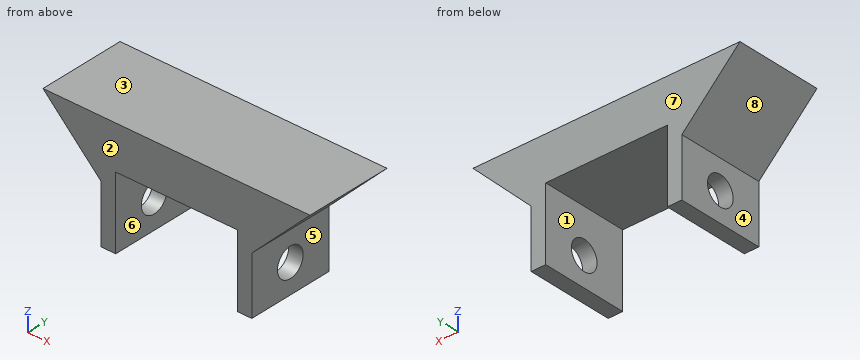
from build123d import *

# Parameters (mm, degrees)
F0_W        = 283.9974
F0_H        = 76.2
F1_DEPTH    = 50.8
F2_T1_DEPTH = 468.124487366
F3_DEPTH    = 50.8
F4_W        = 106.1974
F4_H        = 76.2
F5_DEPTH    = 63.5
F6_R        = 12.7
F7_DEPTH    = 182.3984


# Not quite as in the source:
# - a fillet or chamfer that OpenCascade refuses, or shapes differently, is made with other operations: its cross-section is extruded or revolved along the edge and cut away or added


with BuildPart() as f1:
    # F0 (on Top) → F1 (new body)
    with BuildSketch(Plane.XY):
        with Locations((141.9987, 38.1)):
            Rectangle(F0_W, F0_H)
    extrude(amount=-F1_DEPTH)

    # F2: chamfer of 76.2 on 2 edges, made by hand

    # F2_s2 → F2_t1 (cut)
    with BuildSketch(Plane.XZ.offset(-272.162243683)):
        Polygon((0, 25.4), (76.2, -50.8), (0, -50.8), align=None)
        Polygon((283.9974, 25.4), (207.7974, -50.8), (283.9974, -50.8), align=None)
    extrude(amount=F2_T1_DEPTH, mode=Mode.SUBTRACT)

    # F3 (add): a face of the model
    f3_faces = [f1.faces().sort_by_distance(p)[0] for p in [
        (141.9987, 38.1, -50.8),
    ]]
    extrude(f3_faces, amount=F3_DEPTH)

    # F4 (on face) → F5 (cut)
    with BuildSketch(Plane(origin=(0, 0, -101.6), x_dir=(1, 0, 0), z_dir=(0, 0, -1))):
        with Locations((141.9987, -38.1)):
            Rectangle(F4_W, F4_H)
    extrude(amount=-F5_DEPTH, mode=Mode.SUBTRACT)

    # F6 (on face) → F7 (cut, through all)
    with BuildSketch(Plane.YZ.offset(207.7974)):
        with Locations((38.1, -76.2)):
            Circle(F6_R)
    extrude(amount=-F7_DEPTH, mode=Mode.SUBTRACT)


solid = f1.part
Could you check a few things on this model? Use its own coordinates, in mm. Face numbers are marked on the shaded views. A direction names the side the tool comes from. Give positions to 0.01 mm unless a question says otherwise; leave off trailing zeros. Order: outer loops, then holes, each group sorted by start corner. A loop starts at its lowest first (then second) coordinate and runs counter-clockwise, first axis right, second up. Notation, with made-up numbers: (-26, -23.5) -> (-9, -23.5) arc R24 cw to (-9, 15.5) -> close; hole circle Ø8 at (20.5, 77.5). An arc over 180 degrees is marked (long way). Answer in a Markdown table with one row per item. Add a question column.
Item 1: For the marked faces 1, 2, 3, 4 and 5, which set-ups out of +Z, -Z, +X, -X, +Y, -Y let a thin tool reach every point of the face, with its end or its side?
Item 2: I'm going to push flat-ended pins straight in: P1, Ø6, axis at x = 100, y = 46, coming from the -Z side; P2, Ø4, axis at y = 56.5, z = -21, coming from the +X side; P3, Ø15, axis at y = 38.1, z = -76.2, coming from the +X side; P4, Ø15, axis at y = 52, z = -87.5, coming from the +X side. Where does each tip first touch, or does it pass through?
Item 3: Imagine slicing it at C-C (z = -76.2). List the corners of the cut face in (x, y) for me.
Item 4: Imagine slicing it at A-A (y = 38.1). List the corners of the cut face in (x, z) for me.
Item 5: Imagine slicing it at D-D (y = 11). List the corners of the cut face in (x, z) for me.
Item 6: Please list where these lines run through material, in increasing order: probe 1 along X at (y, z) = (42.5, -89); probe 2 along Z at (x, y) = (199, 38); probe 3 along Y at (x, z) = (80, -76).
Item 7: We'd pull the mould along X, two halves only. Please class the marked faces 6, 7 and 8: pulls with the +X half, pulls with the -X half, needs draft (parallel to the pull), parting line crosses it, or undercut.
Item 8: Imagine slicing it at B-B (z = -57). List the corners of the cut face in (x, y) for me, and give its area (3 significant figures).
Result:
| question | item | result |
|---|---|---|
| 1 | face 1 | -Z, +Y, -Y |
| 1 | face 2 | +Z, -Z, +X, -X, -Y |
| 1 | face 3 | +Z, +X, -X, +Y, -Y |
| 1 | face 4 | -Z, -X, +Y, -Y |
| 1 | face 5 | -Z, +X, +Y, -Y |
| 2 | P1 | z = -38.1 |
| 2 | P2 | x = 239.6 |
| 2 | P3 | through |
| 2 | P4 | x = 207.8 |
| 3 | outline | (76.2, 0) -> (88.9, 0) -> (88.9, 25.4) -> (76.2, 25.4) -> close; (76.2, 50.8) -> (88.9, 50.8) -> (88.9, 76.2) -> (76.2, 76.2) -> close; (195.1, 0) -> (207.8, 0) -> (207.8, 25.4) -> (195.1, 25.4) -> close; (195.1, 50.8) -> (207.8, 50.8) -> (207.8, 76.2) -> (195.1, 76.2) -> close |
| 4 | outline | (25.4, 0) -> (76.2, -50.8) -> (76.2, -63.5) -> (88.9, -63.5) -> (88.9, -38.1) -> (195.1, -38.1) -> (195.1, -63.5) -> (207.8, -63.5) -> (207.8, -50.8) -> (258.6, 0) -> close; (76.2, -101.6) -> (88.9, -101.6) -> (88.9, -88.9) -> (76.2, -88.9) -> close; (195.1, -101.6) -> (207.8, -101.6) -> (207.8, -88.9) -> (195.1, -88.9) -> close |
| 5 | outline | (25.4, 0) -> (76.2, -50.8) -> (76.2, -101.6) -> (88.9, -101.6) -> (88.9, -38.1) -> (195.1, -38.1) -> (195.1, -101.6) -> (207.8, -101.6) -> (207.8, -50.8) -> (258.6, 0) -> close |
| 6 | probe 1 | 76.2 to 88.9, 195.1 to 207.8 |
| 6 | probe 2 | -101.6 to -88.9, -63.5 to 0 |
| 6 | probe 3 | 0 to 25.4, 50.8 to 76.2 |
| 7 | face 6 | undercut |
| 7 | face 7 | needs draft |
| 7 | face 8 | pulls with the -X half |
| 8 | outline | (76.2, 0) -> (88.9, 0) -> (88.9, 76.2) -> (76.2, 76.2) -> close; (195.1, 0) -> (207.8, 0) -> (207.8, 76.2) -> (195.1, 76.2) -> close |
| 8 | area | 1,940 mm2 |
